Part print with two shaded views. Sizes in mm from the minimum x, y, z corner. Coordinates: 2 decimals unless noted, no trailing zeros. Write each loop counter-clockwise with the first axis right and the second up, starting at its lowest first coordinate (ties: lowest second). Pieces come first, ordered by that corner, then holes.
Q1. Pull direction Z, two halves, no side cores. Call the marked faces 1, 2 and 3: released by +Z, released by -Z, zero draft, split by the parting line, or undercut.
Q2. Band-saw the part on A-A, the plane z = 12.7. Write the cut outline in (x, y).
Q3. Band-saw the part on C-C, the plane y = 9.25. Write the cut outline in (x, z), plus the area to 3 significant figures.
Q4. Drill centre lines: probe 1 along Z at (x, y) = (12.7, 6.5); probe 2 along Z at (x, y) = (15.75, 4). Where is each one in solid material? Low to high.
Q5. Band-saw the part on B-B, the plane x = 12.7. Write the cut outline in (y, z).
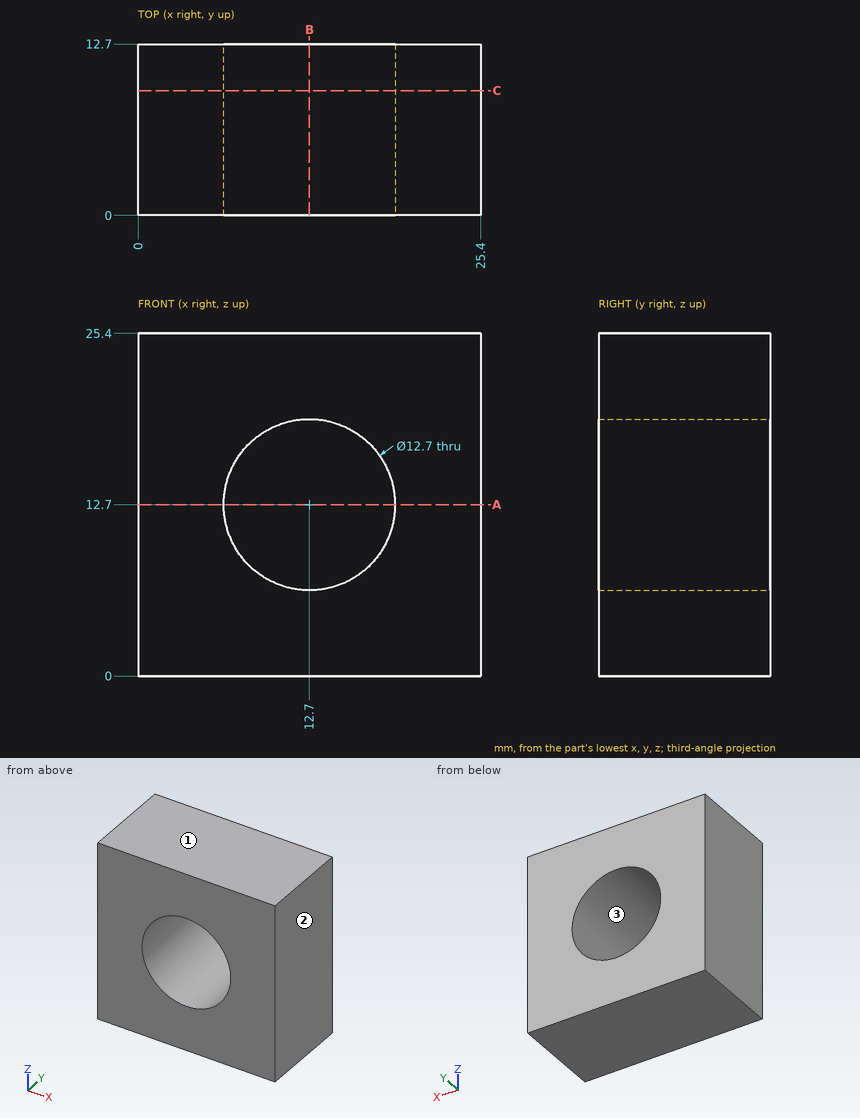
Answer sheet:
1. face 1: released by +Z
1. face 2: zero draft
1. face 3: undercut
2. outline: (0, 0) - (6.35, 0) - (6.35, 12.7) - (0, 12.7) - close; (19.05, 0) - (25.4, 0) - (25.4, 12.7) - (19.05, 12.7) - close
3. outline: (0, 0) - (25.4, 0) - (25.4, 25.4) - (0, 25.4) - close; hole circle Ø12.7 at (12.7, 12.7)
3. area: 518 mm2
4. probe 1: z = 0 to 6.35, 19.05 to 25.4
4. probe 2: z = 0 to 7.13, 18.27 to 25.4
5. outline: (0, 0) - (12.7, 0) - (12.7, 6.35) - (0, 6.35) - close; (0, 19.05) - (12.7, 19.05) - (12.7, 25.4) - (0, 25.4) - close
